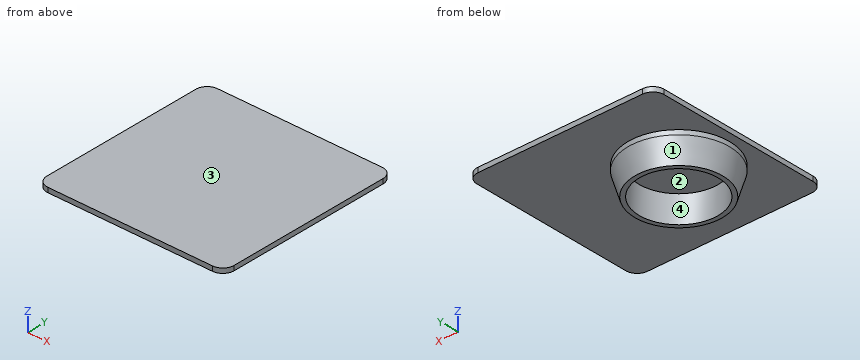
```python
from build123d import *

# Parameters (mm, degrees)
F0_R     = 22.5
F0_R_2   = 17.5
F1_DEPTH = 12
F2_SIZE2 = 3.0573068146
F2_SIZE  = 10
F4_W     = 83
F4_H     = 83
F5_DEPTH = 2.1
F6_R     = 5


with BuildPart() as f1:
    # F0 (on Top) → F1 (new body)
    with BuildSketch(Plane.XY):
        Circle(F0_R)
        Circle(F0_R_2, mode=Mode.SUBTRACT)
    extrude(amount=F1_DEPTH)

    # F2
    f2_edges = [f1.edges().sort_by_distance(p)[0] for p in [
        (-22.5, 0, 0),
    ]]
    f2_side = f1.faces().sort_by_distance((-22.5, 0, 6))[0]
    chamfer(f2_edges, length=F2_SIZE, length2=F2_SIZE2, reference=f2_side)

    # F4 (on offset) → F5 (join)
    with BuildSketch(Plane.XY.offset(14.1)):
        with Locations((15.3470120901, -0.4123098433)):
            Rectangle(F4_W, F4_H)
    extrude(amount=-F5_DEPTH)

    # F6
    f6_edges = [f1.edges().sort_by_distance(p)[0] for p in [
        (-26.152988, -41.91231, 13.05),
        (56.847012, -41.91231, 13.05),
        (-26.152988, 41.08769, 13.05),
        (56.847012, 41.08769, 13.05),
    ]]
    fillet(f6_edges, radius=F6_R)


solid = f1.part
```
Read the model definition and answer for the solid it produces. Units are mm, in the model's axes. Face numbers are marked on the shaded views. Coordinates: 2 decimals unless noted, no trailing zeros. Loops run counter-clockwise (first coordinate to the right, second up) from the corner with the lowest first, then second, coordinate; pieces in that order, holes last. Notation, with made-up numbers: (84, -34.5) - (109, -34.5) arc R30 cw to (109, 3.5) - close; hole circle Ø8 at (-37, 86.5). An arc over 180 degrees is marked (long way). Answer in a Markdown table with one row per item.
1. Given pin 1 (6 mm diameter, centred on x = 30.5, z = 7, fed in from -Y); pin 2 (5 mm diameter, centred on x = -16.5, z = 2, fed in from +Y); pin 3 (2 mm diameter, centred on x = 15.5, z = 7, fed in from +Y); pin 4 (6 mm diameter, centred on x = 14, y = 27.5, fed in from -Z), each flat-ended and moving along its own axis, determine where each tip first touches the part or whether it passes through.
Conclusion:
| item | result |
|---|---|
| pin 1 | passes through |
| pin 2 | stops at y = 14.58 |
| pin 3 | stops at y = 16.08 |
| pin 4 | stops at z = 12 |
2. Find section D-D, the plane x = 41.5. Write down the section's boundary in (y, z).
Conclusion:
| item | result |
|---|---|
| outline | (-41.91, 12) - (41.09, 12) - (41.09, 14.1) - (-41.91, 14.1) - close |
3. Determine the mould class of the marked faces 1, 2, 3 and 4 for opening direction Y: +Y half, -Y half, draft (parallel to the pull), parting line (faces both ways), or undercut.
Conclusion:
| item | result |
|---|---|
| face 1 | parting line |
| face 2 | undercut |
| face 3 | draft |
| face 4 | undercut |
4. Straight lines are drawn through the part: line 1 (Z direction, x = 16, y = 7); line 2 (Y direction, x = -11.5, z = 6.75); line 3 (Y direction, x = 0, z = 5.75). For each, find the intervals that lie inside material, in ascending order.
Conclusion:
| item | result |
|---|---|
| line 1 | z = 12 to 14.1 |
| line 2 | y = -18.17 to -13.19, 13.19 to 18.17 |
| line 3 | y = -21.2 to -17.5, 17.5 to 21.2 |
5. Find section A-A, the plane x = 0. Write down the section's boundary in (y, z), then the cut area to 3 significant figures.
Conclusion:
| item | result |
|---|---|
| outline | (-41.91, 12) - (-22.5, 12) - (-22.5, 10) - (-19.44, 0) - (-17.5, 0) - (-17.5, 12) - (17.5, 12) - (17.5, 0) - (19.44, 0) - (22.5, 10) - (22.5, 12) - (41.09, 12) - (41.09, 14.1) - (-41.91, 14.1) - close |
| area | 264 mm² |
6. Find section C-C, the plane z = 11. Write down the section's boundary in (x, y).
Conclusion:
| item | result |
|---|---|
| outline | circle Ø45 at (0, 0); hole circle Ø35 at (0, 0) |
7. Find section B-B, the plane y = 0. Write down the section's boundary in (x, z).
Conclusion:
| item | result |
|---|---|
| outline | (-26.15, 12) - (-22.5, 12) - (-22.5, 10) - (-19.44, 0) - (-17.5, 0) - (-17.5, 12) - (17.5, 12) - (17.5, 0) - (19.44, 0) - (22.5, 10) - (22.5, 12) - (56.85, 12) - (56.85, 14.1) - (-26.15, 14.1) - close |
